Geometry check sheet. Reference: the model listing, model coordinates, mm. A direction names the side the tool comes from. Coordinates: 2 decimals unless noted, no trailing zeros. Order: outer loops, then holes, each group sorted by start corner. A loop starts at its lowest first (then second) coordinate and runs counter-clockwise, first axis right, second up. Notation, with made-up numbers: (59.25, 24.5) - (89.25, 24.5) arc R21 cw to (89.25, 51.5) - close; hole circle Ø9 at (59, -40). An arc over 180 degrees is marked (long way). Put each result on its own line as item: value.
from build123d import *

# Parameters (mm, degrees)
F0_W     = 215
F0_H     = 215
F1_DEPTH = 600
F2_T     = -20
F4_DEPTH = 20


with BuildPart() as f1:
    # F0 (on Front) → F1 (new body)
    with BuildSketch(Plane.XZ):
        Rectangle(F0_W, F0_H)
    extrude(amount=F1_DEPTH)

    # F2
    f2_openings = [f1.faces().sort_by_distance(p)[0] for p in [
        (0, -300, 107.5),
    ]]
    offset(amount=F2_T, openings=f2_openings)

    # F3 (on face) → F4 (cut, through all)
    with BuildSketch(Plane.XZ.offset(600)):
        with BuildLine():
            Line((-40, -10), (40, -10))
            ThreePointArc((40, -10), (50, 0), (40, 10))
            Line((40, 10), (-40, 10))
            ThreePointArc((-40, 10), (-50, 0), (-40, -10))
        make_face()
    extrude(amount=-F4_DEPTH, mode=Mode.SUBTRACT)


solid = f1.part
Q1. Section check A-A on x = -11.5. Record the boundary of the cut face in (y, z).
Answer block:
outline: (-600, -107.5) - (0, -107.5) - (0, 107.5) - (-20, 107.5) - (-20, -87.5) - (-580, -87.5) - (-580, -10) - (-600, -10) - close; (-600, 10) - (-580, 10) - (-580, 107.5) - (-600, 107.5) - close
Q2. Section check C-C on y = -386.5. Record the boundary of the cut face in (x, z).
Answer block:
outline: (-107.5, -107.5) - (107.5, -107.5) - (107.5, 107.5) - (87.5, 107.5) - (87.5, -87.5) - (-87.5, -87.5) - (-87.5, 107.5) - (-107.5, 107.5) - close
Q3. Thickness scan on L1, parallel to Y at x = 37, z = -49; L2, parallel to X at y = -258.5, z = 0.5; L3, parallel to Z at x = 59, y = -235. Record the ranges inside material, lowest first. Write a range as [from, to].
Answer block:
L1: y = [-600, -580], [-20, 0]
L2: x = [-107.5, -87.5], [87.5, 107.5]
L3: z = [-107.5, -87.5]
Q4. Access from +Z, -Z, +X, -X, +Y, -Y to the whole of each face (thin tool, end or side, straight path). Record for faces 4 (the flat face through (1, -590, 10)), 5 (the flat face through (107.5, -296, -2)), 6 (the flat face through (-87.5, -296, 9)).
Answer block:
face 4: -Y
face 5: +Z, -Z, +X, +Y, -Y
face 6: +Z
Q5. Section check B-B on z = 17.5. Record the boundary of the cut face in (x, y), then the cut area to 3 significant figures.
Answer block:
outline: (-107.5, -600) - (107.5, -600) - (107.5, 0) - (-107.5, 0) - close; hole (-87.5, -580) - (87.5, -580) - (87.5, -20) - (-87.5, -20) - close
area: 31,000 mm^2
Q6. Depth check by flat-ended pin: pin 1 Ø1 at (x, y) = (77, -357.5) entering from +Z; pin 2 Ø1.5 at (x, z) = (-80, 70.5) entering from +Y. Enter the tip coordinate at first touch or a pass-through.
Answer block:
pin 1: stops at z = -87.5
pin 2: stops at y = 0
Q7. Section check D-D on x = 79. Record the boundary of the cut face in (y, z).
Answer block:
outline: (-600, -107.5) - (0, -107.5) - (0, 107.5) - (-20, 107.5) - (-20, -87.5) - (-580, -87.5) - (-580, 107.5) - (-600, 107.5) - close
Q8. Draft check along Y on faces 1 (the flat face through (87.5, -296, 9)), 2 (the flat face through (-1, -590, -10)), 3 (the flat face through (-2, -600, 25)). Enter one of: pulls with the +Y half, pulls with the -Y half, needs draft (parallel to the pull), parting line crosses it, or undercut.
Answer block:
face 1: undercut
face 2: needs draft
face 3: pulls with the -Y half
